For this review, use the dimensioned drawing (mm, ordinates from the lowest corner) and the shaded views. Give positions to 0.01 mm unless a question says otherwise; leave off trailing zeros. Write each loop counter-clockwise with the first axis right and the second up, starting at its lowest first coordinate (ties: lowest second). Pieces come first, ordered by that corner, then holes. Notation, with made-up numbers: M 11.25,74.25 L 48.25,74.25 A14 ccw 48.25,84.25 Z; hole C -22.75,49.5 d6. An arc over 180 degrees is marked long. One line per item, written item: value. Start each with the question number.
Item 1: Mouldability with a two-part tool opening along Y and no side actions: class the marked faces 1, 2 and 3 as released by +Y, released by -Y, zero draft, split by the parting line, or undercut.
Item 2: Clearance check with a flat-ended pin moving along its axis: pin 1 Ø2 at (x, z) = (125.5, 11) entering from -Y. State where the tip first meets the part, or that it passes through.
Item 3: Consider section C-C, the plane z = 13.25. Write out the cut boundary in (x, y), and give its area (3 significant figures).
Item 4: Consider section A-A, the plane x = 100. Write out the cut boundary in (y, z), and give its area (3 significant figures).
Item 5: To check wall thickness, follow probe 1 along Y at (x, z) = (100, 14); probe 2 along X at (y, z) = (69, 5.75); probe 3 along Y at (x, z) = (90, 8). State the ranges of each line that lie inside material, in increasing order.
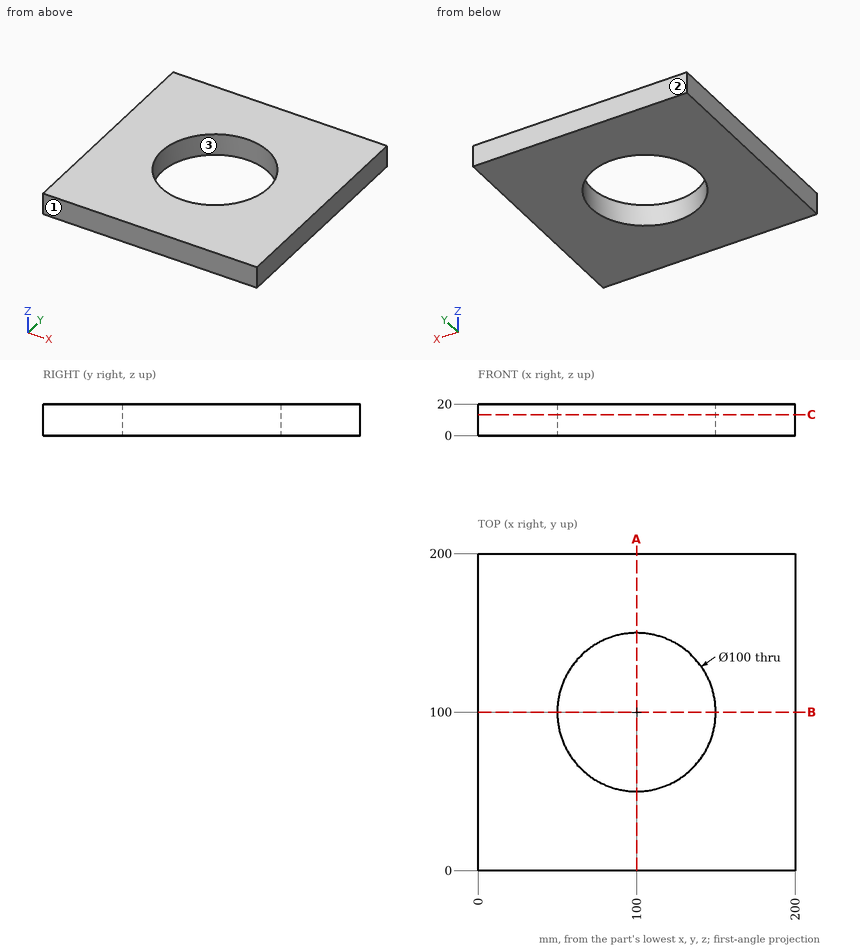
Model answer:
1. face 1: released by -Y
1. face 2: released by +Y
1. face 3: undercut
2. pin 1: stops at y = 0
3. outline: M 0,0 L 200,0 L 200,200 L 0,200 Z; hole C 100,100 d100
3. area: 32,100 mm2
4. outline: M 0,0 L 50,0 L 50,20 L 0,20 Z; M 150,0 L 200,0 L 200,20 L 150,20 Z
4. area: 2,000 mm2
5. probe 1: y = 0 to 50, 150 to 200
5. probe 2: x = 0 to 60.77, 139.23 to 200
5. probe 3: y = 0 to 51.01, 148.99 to 200
